from build123d import *

# Parameters (mm, degrees)
F0_W     = 40
F0_H     = 7
F1_DEPTH = 90
F4_D     = 10
F5_W     = 6
F5_H     = 30
F5_H_2   = 200
F6_DEPTH = 15
F7_DEPTH = 15


# Not quite as in the source:
# - a feature names something its author has since deleted; it is built from what else it names


with BuildPart() as f1:
    # F0 (on Right) → F1 (new body)
    with BuildSketch(Plane.YZ):
        with Locations((0, 3.5)):
            Rectangle(F0_W, F0_H)
    extrude(amount=F1_DEPTH)

    # F4 (through all)
    with Locations(Plane(origin=(0, 0, 0), x_dir=(1, 0, 0), z_dir=(0, 0, -1))):
        with Locations((13, 0), (77, 0)):
            Hole(F4_D / 2)

    # F5 (on Front) → F6 (join)
    with BuildSketch(Plane.XZ):
        with Locations((59.5, 230)):
            Rectangle(F5_W, F5_H)
        Polygon((56.5, 215), (55.5, 200), (61.5, 200), (62.5, 215), align=None)
        with Locations((58.5, 100)):
            Rectangle(F5_W, F5_H_2)
        with Locations((31.5, 100)):
            Rectangle(F5_W, F5_H_2)
        Polygon((27.5, 215), (28.5, 200), (34.5, 200), (33.5, 215), align=None)
        with Locations((30.5, 230)):
            Rectangle(F5_W, F5_H)
    extrude(amount=F6_DEPTH)

    # F7 (add): faces of the model
    f7_faces = [f1.faces().sort_by_distance(p)[0] for p in [
        (31.3424369748, 0, 126),
        (58.6575630252, 0, 126),
    ]]
    extrude(f7_faces, amount=F7_DEPTH)


solid = f1.part
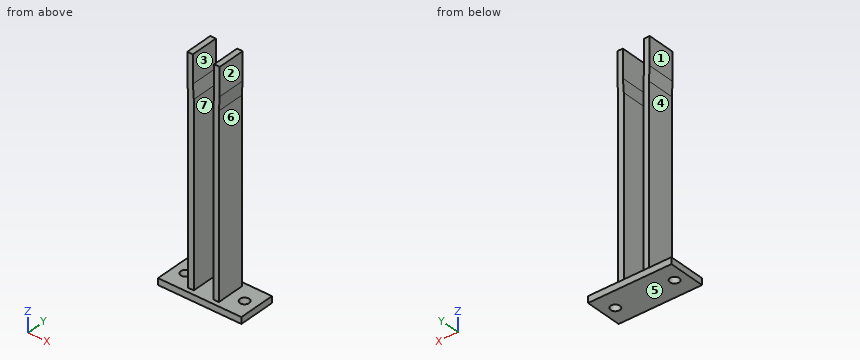
Source: CAD feature listing. Evaluate the final solid. Frame: model axes, mm. Face numbers are marked on the shaded views. A direction names the side the tool comes from. Give positions to 0.01 mm unless a question says otherwise; leave off trailing zeros. Loops run counter-clockwise (first coordinate to the right, second up) from the corner with the lowest first, then second, coordinate; pieces in that order, holes last. Notation, with made-up numbers: (-36.5, 8) -> (22.5, 8) arc R10 cw to (22.5, 12) -> close; hole circle Ø5 at (70.5, -32). An arc over 180 degrees is marked (long way). Use a Markdown table: item, result. Add a question column.
1) Section query D-D, the plane y = 12. Return the cut outline in (x, z), then the cut area to 3 significant figures.
2) Pull-direction query (Z, two-part tool) for the marked faces 4, 5, 6 and 7; classes: +Z half, -Z half, draft (parallel to the pull), parting line (faces both ways), or undercut.
3) Line query: line 1 along X through (y, z) = (13.5, 150); line 2 along Y through (x, z) = (77, 3.5); line 3 along X through (y, z) = (-2.5, 215). Output: solid intervals per line, ascending. Write a range as [from, to].
4) Section query B-B, the plane y = 0. Return the cut outline in (x, z), then the cut area to 3 significant figures.
5) Section query A-A, the plane z = 176. Return the cut outline in (x, y).
6) First-contact query: pin 1 (15 mm diameter, centred on y = -1.5, z = 113.5, fed in from -X); pin 2 (1.5 mm diameter, centred on x = 61.5, z = 43.5, fed in from +Y); pin 3 (3.5 mm diameter, centred on x = 32, z = 125, fed in from -Y). Flat tips, straight axial feed; report the tip coordinate or a pass-through.
7) Section query C-C, the plane x = 13. Return the cut outline in (y, z).
8) Reachability of the marked faces 1, 2 and 3 from +Z, -Z, +X, -X, +Y, -Y: full face, straight path, thin tool, end or side. Return the list, or none.
Numbers:
| question | item | result |
|---|---|---|
| 1 | outline | (0, 0) -> (90, 0) -> (90, 7) -> (61.5, 7) -> (61.5, 200) -> (62.5, 215) -> (62.5, 245) -> (56.5, 245) -> (56.5, 215) -> (55.5, 200) -> (55.5, 7) -> (34.5, 7) -> (34.5, 200) -> (33.5, 215) -> (33.5, 245) -> (27.5, 245) -> (27.5, 215) -> (28.5, 200) -> (28.5, 7) -> (0, 7) -> close |
| 1 | area | 3,490 mm2 |
| 2 | face 4 | undercut |
| 2 | face 5 | -Z half |
| 2 | face 6 | undercut |
| 2 | face 7 | draft |
| 3 | line 1 | x = [28.5, 34.5], [55.5, 61.5] |
| 3 | line 2 | y = [-20, -5], [5, 20] |
| 3 | line 3 | x = [27.5, 33.5], [56.5, 62.5] |
| 4 | outline | (0, 0) -> (8, 0) -> (8, 7) -> (0, 7) -> close; (18, 0) -> (72, 0) -> (72, 7) -> (61.5, 7) -> (61.5, 200) -> (62.5, 215) -> (62.5, 245) -> (56.5, 245) -> (56.5, 215) -> (55.5, 200) -> (55.5, 7) -> (34.5, 7) -> (34.5, 200) -> (33.5, 215) -> (33.5, 245) -> (27.5, 245) -> (27.5, 215) -> (28.5, 200) -> (28.5, 7) -> (18, 7) -> close; (82, 0) -> (90, 0) -> (90, 7) -> (82, 7) -> close |
| 4 | area | 3,350 mm2 |
| 5 | outline | (28.5, -15) -> (34.5, -15) -> (34.5, 15) -> (28.5, 15) -> close; (55.5, -15) -> (61.5, -15) -> (61.5, 15) -> (55.5, 15) -> close |
| 6 | pin 1 | stops at x = 28.5 |
| 6 | pin 2 | stops at y = 15 |
| 6 | pin 3 | stops at y = -15 |
| 7 | outline | (-20, 0) -> (-5, 0) -> (-5, 7) -> (-20, 7) -> close; (5, 0) -> (20, 0) -> (20, 7) -> (5, 7) -> close |
| 8 | face 1 | +Z, -X, +Y, -Y |
| 8 | face 2 | +Z, +X, +Y, -Y |
| 8 | face 3 | +Z, +Y, -Y |
